from build123d import *

# Parameters (mm, degrees)
SKETCH_1_R      = 1.1
SKETCH_1_R_2    = 1.35
EXTRUDE_1_DEPTH = 2


with BuildPart() as part:
    # 草图1 → 凸台-拉伸1 (new body)
    with BuildSketch(Plane.XY):
        with BuildLine():
            Line((36.2, 20.95), (36.2, 1.75))
            ThreePointArc((36.2, 1.75), (36.346446609, 1.396446609), (36.7, 1.25))
            ThreePointArc((36.7, 1.25), (37.053553391, 1.103553391), (37.2, 0.75))
            Line((37.2, 0.75), (37.2, -1.631966011))
            ThreePointArc((37.2, -1.631966011), (37.186624495, -1.746842472), (37.147213595, -1.855572809))
            Line((37.147213595, -1.855572809), (36.338196601, -3.473606798))
            ThreePointArc((36.338196601, -3.473606798), (36.153848562, -3.675325404), (35.890983006, -3.75))
            Line((35.890983006, -3.75), (35.2, -3.75))
            ThreePointArc((35.2, -3.75), (34.846446609, -3.603553391), (34.7, -3.25))
            Line((34.7, -3.25), (34.7, -2.25))
            ThreePointArc((34.7, -2.25), (34.553553391, -1.896446609), (34.2, -1.75))
            Line((34.2, -1.75), (28.75, -1.75))
            ThreePointArc((28.75, -1.75), (28.431801948, -1.881801948), (28.3, -2.2))
            Line((28.3, -2.2), (28.3, -5.5))
            ThreePointArc((28.3, -5.5), (28.168198052, -5.818198052), (27.85, -5.95))
            Line((27.85, -5.95), (20.75, -5.95))
            ThreePointArc((20.75, -5.95), (20.431801948, -5.818198052), (20.3, -5.5))
            Line((20.3, -5.5), (20.3, -2.2))
            ThreePointArc((20.3, -2.2), (20.168198052, -1.881801948), (19.85, -1.75))
            Line((19.85, -1.75), (16.2, -1.75))
            Line((16.2, -1.75), (16.2, -0.95))
            Line((16.2, -0.95), (1, -0.95))
            Line((1, -0.95), (1, -11.25))
            ThreePointArc((1, -11.25), (1.353553391, -12.103553391), (0.5, -11.75))
            Line((0.5, -11.75), (-0.5, -11.75))
            ThreePointArc((-0.5, -11.75), (-1.353553391, -12.103553391), (-1, -11.25))
            Line((-1, -11.25), (-1, -0.95))
            Line((-1, -0.95), (-16.2, -0.95))
            Line((-16.2, -0.95), (-16.2, -1.75))
            Line((-16.2, -1.75), (-19.85, -1.75))
            ThreePointArc((-19.85, -1.75), (-20.168198052, -1.881801948), (-20.3, -2.2))
            Line((-20.3, -2.2), (-20.3, -5.5))
            ThreePointArc((-20.3, -5.5), (-20.431801948, -5.818198052), (-20.75, -5.95))
            Line((-20.75, -5.95), (-27.85, -5.95))
            ThreePointArc((-27.85, -5.95), (-28.168198052, -5.818198052), (-28.3, -5.5))
            Line((-28.3, -5.5), (-28.3, -2.2))
            ThreePointArc((-28.3, -2.2), (-28.431801948, -1.881801948), (-28.75, -1.75))
            Line((-28.75, -1.75), (-34.2, -1.75))
            ThreePointArc((-34.2, -1.75), (-34.553553391, -1.896446609), (-34.7, -2.25))
            Line((-34.7, -2.25), (-34.7, -3.25))
            ThreePointArc((-34.7, -3.25), (-34.846446609, -3.603553391), (-35.2, -3.75))
            Line((-35.2, -3.75), (-35.890983006, -3.75))
            ThreePointArc((-35.890983006, -3.75), (-36.153848562, -3.675325404), (-36.338196601, -3.473606798))
            Line((-36.338196601, -3.473606798), (-37.147213595, -1.855572809))
            ThreePointArc((-37.147213595, -1.855572809), (-37.186624495, -1.746842472), (-37.2, -1.631966011))
            Line((-37.2, -1.631966011), (-37.2, 0.75))
            ThreePointArc((-37.2, 0.75), (-37.053553391, 1.103553391), (-36.7, 1.25))
            ThreePointArc((-36.7, 1.25), (-36.346446609, 1.396446609), (-36.2, 1.75))
            Line((-36.2, 1.75), (-36.2, 20.95))
            ThreePointArc((-36.2, 20.95), (-36.434314575, 21.515685425), (-37, 21.75))
            Line((-37, 21.75), (-39.671594525, 21.75))
            ThreePointArc((-39.671594525, 21.75), (-41.393669971, 21.407457896), (-42.85357504, 20.431980515))
            Line((-42.85357504, 20.431980515), (-43.685952604, 19.599602951))
            ThreePointArc((-43.685952604, 19.599602951), (-46.725975031, 17.519131379), (-50.31301428, 16.680532699))
            Line((-50.31301428, 16.680532699), (-67, 15.938888889))
            Line((-67, 15.938888889), (-72.978782406, 15.739596142))
            ThreePointArc((-72.978782406, 15.739596142), (-74.349730451, 15.13116321), (-74.912152745, 13.740706328))
            Line((-74.912152745, 13.740706328), (-74.912152745, 3.600025905))
            ThreePointArc((-74.912152745, 3.600025905), (-74.052488898, 0.796881859), (-71.769106127, -1.042357549))
            Line((-71.769106127, -1.042357549), (-20, -21.75))
            Line((-20, -21.75), (20, -21.75))
            Line((20, -21.75), (71.769106127, -1.042357549))
            ThreePointArc((71.769106127, -1.042357549), (74.052488898, 0.796881859), (74.912152745, 3.600025905))
            Line((74.912152745, 3.600025905), (74.912152745, 13.740706328))
            ThreePointArc((74.912152745, 13.740706328), (74.349730451, 15.13116321), (72.978782406, 15.739596142))
            Line((72.978782406, 15.739596142), (67, 15.938888889))
            Line((67, 15.938888889), (50.31301428, 16.680532699))
            ThreePointArc((50.31301428, 16.680532699), (46.725975031, 17.519131379), (43.685952604, 19.599602951))
            Line((43.685952604, 19.599602951), (42.85357504, 20.431980515))
            ThreePointArc((42.85357504, 20.431980515), (41.393669971, 21.407457896), (39.671594525, 21.75))
            Line((39.671594525, 21.75), (37, 21.75))
            ThreePointArc((37, 21.75), (36.434314575, 21.515685425), (36.2, 20.95))
        make_face()
        with Locations((72.75, 3.75716439)):
            Circle(SKETCH_1_R, mode=Mode.SUBTRACT)
        with Locations((72.75, 11.75716439)):
            Circle(SKETCH_1_R, mode=Mode.SUBTRACT)
        with Locations((38.7, 19.25)):
            Circle(SKETCH_1_R, mode=Mode.SUBTRACT)
        with Locations((32.3, -4.25)):
            Circle(SKETCH_1_R, mode=Mode.SUBTRACT)
        with Locations((18.3, -4.25)):
            Circle(SKETCH_1_R, mode=Mode.SUBTRACT)
        with Locations((20, -13.75)):
            Circle(SKETCH_1_R_2, mode=Mode.SUBTRACT)
        with Locations((-18.3, -4.25)):
            Circle(SKETCH_1_R, mode=Mode.SUBTRACT)
        with Locations((-32.3, -4.25)):
            Circle(SKETCH_1_R, mode=Mode.SUBTRACT)
        with Locations((-20, -13.75)):
            Circle(SKETCH_1_R_2, mode=Mode.SUBTRACT)
        with Locations((-38.7, 19.25)):
            Circle(SKETCH_1_R, mode=Mode.SUBTRACT)
        with Locations((-72.75, 3.75716439)):
            Circle(SKETCH_1_R, mode=Mode.SUBTRACT)
        with Locations((-72.75, 11.75716439)):
            Circle(SKETCH_1_R, mode=Mode.SUBTRACT)
    extrude(amount=EXTRUDE_1_DEPTH)


solid = part.part
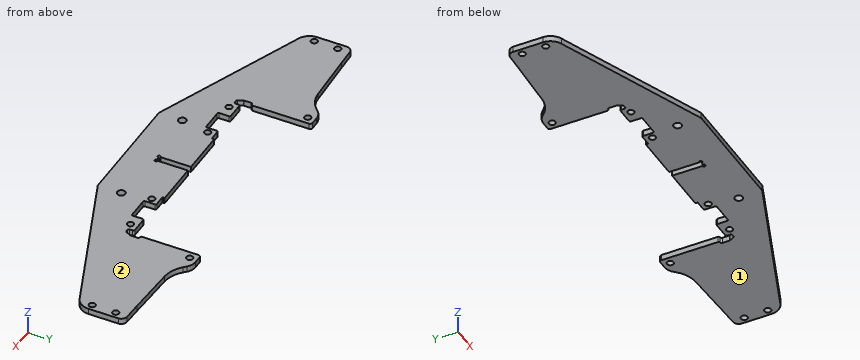
Geometry: final body of the model. Coordinates: model frame, mm. Face numbers are marked on the shaded views. Coordinates: 2 decimals unless noted, no trailing zeros. Loops run counter-clockwise (first coordinate to the right, second up) from the corner with the lowest first, then second, coordinate; pieces in that order, holes last. Notation, with made-up numbers: (19.25, -5.75) - (32.25, -5.75) arc R27 ccw to (32.25, 16.25) - close; hole circle Ø10 at (-30, 54). An arc over 180 degrees is marked (long way). One line per question, with ' | ' between items. Start each with the question number.
(1) Ray query, L1, parallel to X at y = 5, z = 0.3; L2, parallel to X at y = 12, z = 0.95; L3, parallel to Y at x = -18.3, z = 1.45. Return the intervals inside material, ascending. Write a range as from..to.
(2) Draft query along Z for the marked faces 1 and 2. Return one class per face: +Z half, -Z half, draft (parallel to the pull), parting line (faces both ways), or undercut.
(3) Cut plane A-A on y = 9. Output: boundary loops of the cut face in (x, z), and give its area (3 significant figures).
(4) Cut plane C-C on z = 1.45. Count the separate pieces of the cut face and the enclosed holes in it, and give its area (3 significant figures).
(5) Cut plane B-B on x = -4. Output: boundary loops of the cut face in (y, z).
(6) Cut plane D-D on y = -17. Output: boundary loops of the cut face in (x, z) (3 decimals).
(7) First-contact query: pin 1 (1 mm diameter, centred on x = 10.5, z = 1.5, fed in from +Y); pin 2 (0.6 mm diameter, centred on y = -1, z = 1.5, fed in from -X); pin 3 (1.1 mm diameter, centred on y = -3, z = 0.5, fed in from -X). Flat tips, straight axial feed; report the tip coordinate or a pass-through.
Here are the results:
1) L1: -74.91..-36.2, 36.2..74.91 | L2: -74.91..-73.82, -71.68..-36.2, 36.2..71.68, 73.82..74.91 | L3: -21.75..-5.35, -3.15..-1.75
2) face 1: -Z half | face 2: +Z half
3) outline: (-74.91, 0) - (-36.2, 0) - (-36.2, 2) - (-74.91, 2) - close; (36.2, 0) - (74.91, 0) - (74.91, 2) - (36.2, 2) - close | area: 155 mm²
4) separate pieces: 1 | enclosed holes: 12 | area: 3,140 mm²
5) outline: (-21.75, 0) - (-0.95, 0) - (-0.95, 2) - (-21.75, 2) - close
6) outline: (-31.875, 0) - (31.875, 0) - (31.875, 2) - (-31.875, 2) - close
7) pin 1: y = -0.95 | pin 2: x = -72.46 | pin 3: x = -68.25
